Geometry: final body of the model. Coordinates: model frame, mm. A direction names the side the tool comes from. Give positions to 0.01 mm unless a question says otherwise; leave off trailing zeros. Order: outer loops, then holes, each group sorted by start corner. A loop starts at its lowest first (then second) coordinate and runs counter-clockwise, first axis right, second up. Notation, with made-up numbers: (65.25, 37) - (81.25, 37) arc R21 ccw to (81.25, 63) - close; hole circle Ø3 at (-13, 61.5). An arc over 180 degrees is marked (long way). Put each result on its own line as item: value. Start each with the question number.
1. Set-up query: faces 1 (the flat face through (52.265, -50, -9)), 2 (the flat face through (-69.655, -50, -13)). Return all of +Z, -Z, +X, -X, +Y, -Y with unobstructed straight access to the full face (end or side cutting, diameter ignored); none if empty.
2. Section A-A on y = -45.5. Return the cut outline in (x, z), plus the area to 3 significant figures.
3. Section B-B on z = -8. Return the cut outline in (x, y).
4. Section C-C on x = 10. Return the cut outline in (y, z), plus the area to 3 significant figures.
5. Ray query, line 1 along Y through (x, z) = (-16.5, -15.5); line 2 along X through (y, z) = (-29, 9); line 3 along Z through (x, y) = (-53, -7.5). Return the intervals inside material, ascending. Write a range as from..to.
6. Mould query, pull axis X, two halves, no side actions, for faces 3 (the flat face through (57.345, -50, -13)), 4 (the flat face through (-7, 0, -12)), 5 (the flat face through (-7, -96.52, -8)). Classes: pulls with the +X half, pulls with the -X half, needs draft (parallel to the pull), parting line crosses it, or undercut.
7. First-contact query: P1, Ø5, axis at x = 11.5, y = -54, coming from the +Z side. Flat tip, straight axial feed; report the tip coordinate or a pass-through.
from build123d import *

# Parameters (mm, degrees)
F0_W     = 127
F0_H     = 76.2
F1_DEPTH = 101.6
F2_T     = -5.08
F3_R     = 2.54


with BuildPart() as f1:
    # F0 (on Front) → F1 (new body)
    with BuildSketch(Plane.XZ):
        with Locations((-6.154592, -11.322558)):
            Rectangle(F0_W, F0_H)
    extrude(amount=F1_DEPTH)

    # F2
    f2_openings = [f1.faces().sort_by_distance(p)[0] for p in [
        (-6.154592, -50.8, 26.777442),
    ]]
    offset(amount=F2_T, openings=f2_openings)

    # F3
    f3_edges = [f1.edges().sort_by_distance(p)[0] for p in [
        (-6.154592, -101.6, 26.777442),
        (-69.654592, -50.8, 26.777442),
        (-6.154592, 0, 26.777442),
        (57.345408, -50.8, 26.777442),
    ]]
    fillet(f3_edges, radius=F3_R)


solid = f1.part
Resolved:
1. face 1: +Z
1. face 2: +Z, -Z, -X, +Y, -Y
2. outline: (-69.65, -49.42) - (57.35, -49.42) - (57.35, 24.24) arc R2.54 ccw to (54.81, 26.78) - (52.27, 26.78) - (52.27, -44.34) - (-64.57, -44.34) - (-64.57, 26.78) - (-67.11, 26.78) arc R2.54 ccw to (-69.65, 24.24) - close
2. area: 1,360 mm^2
3. outline: (-69.65, -101.6) - (57.35, -101.6) - (57.35, 0) - (-69.65, 0) - close; hole (-64.57, -96.52) - (52.27, -96.52) - (52.27, -5.08) - (-64.57, -5.08) - close
4. outline: (-101.6, -49.42) - (0, -49.42) - (0, 24.24) arc R2.54 ccw to (-2.54, 26.78) - (-5.08, 26.78) - (-5.08, -44.34) - (-96.52, -44.34) - (-96.52, 26.78) - (-99.06, 26.78) arc R2.54 ccw to (-101.6, 24.24) - close
4. area: 1,240 mm^2
5. line 1: -101.6..-96.52, -5.08..0
5. line 2: -69.65..-64.57, 52.27..57.35
5. line 3: -49.42..-44.34
6. face 3: pulls with the +X half
6. face 4: needs draft
6. face 5: undercut
7. P1: z = -44.34
